from build123d import *

# Parameters (mm, degrees)
SKETCH_1_W               = 177
SKETCH_1_H               = 42
SKETCH_1_R               = 1.55
SKETCH_1_R_2             = 13.4
EXTRUDE_1_DEPTH          = 1.5
SKETCH_3_W               = 6.5
SKETCH_3_H               = 20
CUT_EXTRUDE_1_DEPTH      = 4
SKETCH_4_W               = 3.5
SKETCH_4_H               = 7
EXTRUDE_2_DEPTH          = 3
SKETCH_5_R               = 0.75
CUT_EXTRUDE_2_DEPTH      = 4
FILLET_1_R               = 1
SKETCH_6_R               = 1.55
CUT_EXTRUDE_3_DEPTH      = 1
CUT_EXTRUDE_3_DEPTH_BACK = 4
CUT_EXTRUDE_4_DEPTH      = 4
SKETCH_8_W               = 12
SKETCH_8_H               = 18
CUT_EXTRUDE_5_DEPTH      = 4
FILLET_2_R               = 2


with BuildPart() as part:
    # 草图1 → 凸台-拉伸1 (new body, symmetric)
    with BuildSketch(Plane(origin=(0, 0, 0), x_dir=(1, 0, 0), z_dir=(0, 1, 0))):
        Rectangle(SKETCH_1_W, SKETCH_1_H)
        with Locations((-67.5, 17.5)):
            Circle(SKETCH_1_R, mode=Mode.SUBTRACT)
        with Locations((-55.125631329, 12.374368671)):
            Circle(SKETCH_1_R, mode=Mode.SUBTRACT)
        with Locations((-50, 0)):
            Circle(SKETCH_1_R, mode=Mode.SUBTRACT)
        with Locations((-55.125631329, -12.374368671)):
            Circle(SKETCH_1_R, mode=Mode.SUBTRACT)
        with Locations((-67.5, -17.5)):
            Circle(SKETCH_1_R, mode=Mode.SUBTRACT)
        with Locations((-79.874368671, -12.374368671)):
            Circle(SKETCH_1_R, mode=Mode.SUBTRACT)
        with Locations((-85, 0)):
            Circle(SKETCH_1_R, mode=Mode.SUBTRACT)
        with Locations((-79.874368671, 12.374368671)):
            Circle(SKETCH_1_R, mode=Mode.SUBTRACT)
        with Locations((67.5, 17.5)):
            Circle(SKETCH_1_R, mode=Mode.SUBTRACT)
        with Locations((55.125631329, 12.374368671)):
            Circle(SKETCH_1_R, mode=Mode.SUBTRACT)
        with Locations((50, 0)):
            Circle(SKETCH_1_R, mode=Mode.SUBTRACT)
        with Locations((55.125631329, -12.374368671)):
            Circle(SKETCH_1_R, mode=Mode.SUBTRACT)
        with Locations((67.5, -17.5)):
            Circle(SKETCH_1_R, mode=Mode.SUBTRACT)
        with Locations((79.874368671, -12.374368671)):
            Circle(SKETCH_1_R, mode=Mode.SUBTRACT)
        with Locations((85, 0)):
            Circle(SKETCH_1_R, mode=Mode.SUBTRACT)
        with Locations((79.874368671, 12.374368671)):
            Circle(SKETCH_1_R, mode=Mode.SUBTRACT)
        with Locations((-67.5, 0)):
            Circle(SKETCH_1_R_2, mode=Mode.SUBTRACT)
        with Locations((67.5, 0)):
            Circle(SKETCH_1_R_2, mode=Mode.SUBTRACT)
    extrude(amount=EXTRUDE_1_DEPTH, both=True)

    # 草图3 → 切除-拉伸1 (cut, through all)
    with BuildSketch(Plane(origin=(0, 1.5, 0), x_dir=(1, 0, 0), z_dir=(0, 1, 0))):
        with Locations((15.775, 0)):
            Rectangle(SKETCH_3_W, SKETCH_3_H)
        with Locations((-15.775, 0)):
            Rectangle(SKETCH_3_W, SKETCH_3_H)
    extrude(amount=-CUT_EXTRUDE_1_DEPTH, mode=Mode.SUBTRACT)

    # 草图4 → 凸台-拉伸2 (add)
    with BuildSketch(Plane(origin=(0, 1.5, 0), x_dir=(1, 0, 0), z_dir=(0, 1, 0))):
        with Locations((-14.275, 0)):
            Rectangle(SKETCH_4_W, SKETCH_4_H)
        with Locations((14.275, 0)):
            Rectangle(SKETCH_4_W, SKETCH_4_H)
    extrude(amount=-EXTRUDE_2_DEPTH)

    # 草图5 → 切除-拉伸2 (cut, through all)
    with BuildSketch(Plane(origin=(0, 1.5, 0), x_dir=(1, 0, 0), z_dir=(0, 1, 0))):
        with Locations((12.525, 4.25)):
            Circle(SKETCH_5_R)
        with Locations((12.525, -4.25)):
            Circle(SKETCH_5_R)
        with Locations((13.275, -10)):
            Circle(SKETCH_5_R)
        with Locations((13.275, 10)):
            Circle(SKETCH_5_R)
        with Locations((19.025, 9.25)):
            Circle(SKETCH_5_R)
        with Locations((19.025, -9.25)):
            Circle(SKETCH_5_R)
        with Locations((-19.025, -9.25)):
            Circle(SKETCH_5_R)
        with Locations((-19.025, 9.25)):
            Circle(SKETCH_5_R)
        with Locations((-13.275, 10)):
            Circle(SKETCH_5_R)
        with Locations((-13.275, -10)):
            Circle(SKETCH_5_R)
        with Locations((-12.525, -4.25)):
            Circle(SKETCH_5_R)
        with Locations((-12.525, 4.25)):
            Circle(SKETCH_5_R)
    extrude(amount=-CUT_EXTRUDE_2_DEPTH, mode=Mode.SUBTRACT)

    # 圆角1
    fillet_1_edges = [part.edges().sort_by_distance(p)[0] for p in [
        (-16.025, 0, 3.5),
        (-16.025, 0, -3.5),
        (16.025, 0, -3.5),
        (16.025, 0, 3.5),
    ]]
    fillet(fillet_1_edges, radius=FILLET_1_R)

    # 草图6 → 切除-拉伸3 (cut, two sides)
    with BuildSketch(Plane(origin=(0, 1.5, 0), x_dir=(1, 0, 0), z_dir=(0, 1, 0))) as cut_extrude_3_sk:
        with Locations((-32.5, 13.5)):
            Circle(SKETCH_6_R)
        with Locations((-32.5, -13.5)):
            Circle(SKETCH_6_R)
        with Locations((-7.5, 10)):
            Circle(SKETCH_6_R)
        with Locations((-7.5, -10)):
            Circle(SKETCH_6_R)
        with Locations((7.5, -10)):
            Circle(SKETCH_6_R)
        with Locations((7.5, 10)):
            Circle(SKETCH_6_R)
        with Locations((32.5, 13.5)):
            Circle(SKETCH_6_R)
        with Locations((32.5, -13.5)):
            Circle(SKETCH_6_R)
    extrude(amount=CUT_EXTRUDE_3_DEPTH, mode=Mode.SUBTRACT)
    extrude(cut_extrude_3_sk.sketch, amount=-CUT_EXTRUDE_3_DEPTH_BACK, mode=Mode.SUBTRACT)

    # 草图7 → 切除-拉伸4 (cut, through all)
    with BuildSketch(Plane.XZ.offset(1.5)):
        Polygon((-35, 21), (-27.558405496, 14), (27.558405496, 14), (35, 21), align=None)
        Polygon((-88.5, 8.69848481), (-76.19848481, 21), (-88.5, 21), align=None)
        Polygon((76.19848481, 21), (88.5, 21), (88.5, 8.69848481), align=None)
    cut_extrude_4 = extrude(amount=-CUT_EXTRUDE_4_DEPTH, mode=Mode.SUBTRACT)

    # 镜向1: 切除-拉伸4 across plane
    add(cut_extrude_4.mirror(Plane.XY), mode=Mode.SUBTRACT)

    # 草图8 → 切除-拉伸5 (cut, through all)
    with BuildSketch(Plane.XZ.offset(1.5)):
        with Locations((-39, 0)):
            Rectangle(SKETCH_8_W, SKETCH_8_H)
        with Locations((39, 0)):
            Rectangle(SKETCH_8_W, SKETCH_8_H)
    extrude(amount=-CUT_EXTRUDE_5_DEPTH, mode=Mode.SUBTRACT)

    # 圆角2
    fillet_2_edges = [part.edges().sort_by_distance(p)[0] for p in [
        (-45, 0, -9),
        (-45, 0, 9),
        (-33, 0, 9),
        (-33, 0, -9),
        (33, 0, -9),
        (33, 0, 9),
        (45, 0, 9),
        (45, 0, -9),
    ]]
    fillet(fillet_2_edges, radius=FILLET_2_R)


solid = part.part
Read the model definition and answer for the solid it produces. Units are mm, in the model's axes. A direction names the side the tool comes from. Coordinates: 2 decimals unless noted, no trailing zeros. Loops run counter-clockwise (first coordinate to the right, second up) from the corner with the lowest first, then second, coordinate; pieces in that order, holes last. Notation, with made-up numbers: (59, -5) -> (66, -5) arc R16 cw to (66, 2) -> close; hole circle Ø10 at (41.25, 54). An arc over 180 degrees is marked (long way). Answer in a Markdown table with one row per item.
Item 1: For a pull along Z with two mould halves and no side action, classify faces 1 (the flat face through (-1, 1.5, 0)), 2 (the flat face through (33, 0, 0)), 3 (the flat face through (0, 0, -14)) as released by +Z, released by -Z, zero draft, split by the parting line, or undercut.
Returned:
| item | result |
|---|---|
| face 1 | zero draft |
| face 2 | undercut |
| face 3 | released by -Z |
Item 2: For faces 4 (the flat face through (16.025, 0, 0)), 5 (the flat face through (-82.4, 0, -14.8)), determine the directions among +Z, -Z, +X, -X, +Y, -Y from which every point of the face is accessible in a straight line to the end or side of a thin tool.
Returned:
| item | result |
|---|---|
| face 4 | +Y, -Y |
| face 5 | -Z, -X, +Y, -Y |
Item 3: Straight lines are drawn through the part: line 1 along Z through (x, y) = (-7.5, -0.6); line 2 along Z through (x, y) = (37, 0.45); line 3 along Z through (x, y) = (-32.5, -0.7). For each, find the intervals that lie inside material, in ascending order. Write a range as [from, to].
Returned:
| item | result |
|---|---|
| line 1 | z = [-14, -11.55], [-8.45, 8.45], [11.55, 14] |
| line 2 | z = [-21, -9], [9, 21] |
| line 3 | z = [-18.65, -15.05], [-11.95, 11.95], [15.05, 18.65] |
Item 4: Each of these flat-tipped pins is pushed along its axis until it touches: P1, Ø0.9, axis at x = 6, y = 0, coming from the -Z side; P2, Ø5, axis at x = 32.5, z = 13.5, coming from the +Y side; P3, Ø2.5, axis at x = 67.5, z = -17.5, coming from the +Y side; P4, Ø1.5, axis at x = -18.5, y = 0, coming from the +Z side. Where does it stop, or does it pass through?
Returned:
| item | result |
|---|---|
| P1 | stops at z = -14 |
| P2 | stops at y = 1.5 |
| P3 | passes through |
| P4 | stops at z = 14 |
Item 5: A cutting plane is placed at B-B on x = -67.5. Determine the outline of the cut face in (y, z).
Returned:
| item | result |
|---|---|
| outline | (-1.5, -21) -> (1.5, -21) -> (1.5, -19.05) -> (-1.5, -19.05) -> close; (-1.5, -15.95) -> (1.5, -15.95) -> (1.5, -13.4) -> (-1.5, -13.4) -> close; (-1.5, 13.4) -> (1.5, 13.4) -> (1.5, 15.95) -> (-1.5, 15.95) -> close; (-1.5, 19.05) -> (1.5, 19.05) -> (1.5, 21) -> (-1.5, 21) -> close |
Item 6: A cutting plane is placed at D-D on x = 62.5. Determine the outline of the cut face in (y, z).
Returned:
| item | result |
|---|---|
| outline | (-1.5, -21) -> (1.5, -21) -> (1.5, -12.43) -> (-1.5, -12.43) -> close; (-1.5, 12.43) -> (1.5, 12.43) -> (1.5, 21) -> (-1.5, 21) -> close |
Item 7: A cutting plane is placed at C-C on z = -17.5. Determine the outline of the cut face in (x, y).
Returned:
| item | result |
|---|---|
| outline | (-79.7, -1.5) -> (-69.05, -1.5) -> (-69.05, 1.5) -> (-79.7, 1.5) -> close; (-65.95, -1.5) -> (-31.28, -1.5) -> (-31.28, 1.5) -> (-65.95, 1.5) -> close; (31.28, -1.5) -> (65.95, -1.5) -> (65.95, 1.5) -> (31.28, 1.5) -> close; (69.05, -1.5) -> (79.7, -1.5) -> (79.7, 1.5) -> (69.05, 1.5) -> close |
Item 8: A cutting plane is placed at A-A on x = -7.5. Determine the outline of the cut face in (y, z).
Returned:
| item | result |
|---|---|
| outline | (-1.5, -14) -> (1.5, -14) -> (1.5, -11.55) -> (-1.5, -11.55) -> close; (-1.5, -8.45) -> (1.5, -8.45) -> (1.5, 8.45) -> (-1.5, 8.45) -> close; (-1.5, 11.55) -> (1.5, 11.55) -> (1.5, 14) -> (-1.5, 14) -> close |
